Build history of the part. All positions in model axes, mm. Face numbers are marked on the shaded views. A direction names the side the tool comes from. Give positions to 0.01 mm unless a question says otherwise; leave off trailing zeros. Order: outer loops, then holes, each group sorted by start corner. A loop starts at its lowest first (then second) coordinate and runs counter-clockwise, first axis right, second up. Notation, with made-up numbers: (25.5, -31) - (77.5, -31) arc R17 ccw to (77.5, -26) - close; hole circle Ø5 at (19.25, 45.25). An arc over 180 degrees is marked (long way). Use a Markdown table: item, result.
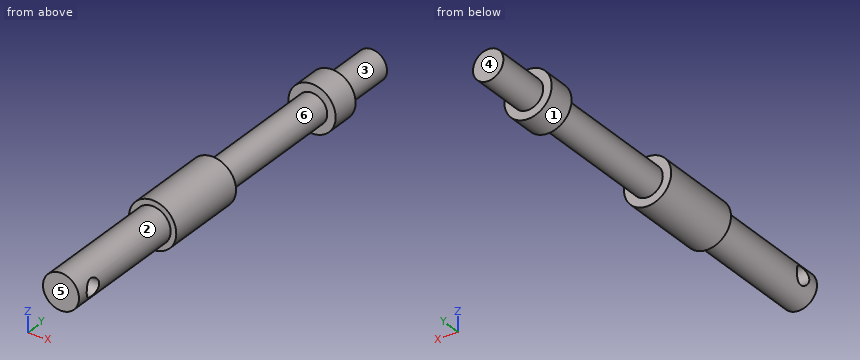
Autodesk Inventor part; units mm, degrees
ref_plane "YZ Plane" through (0, 0, 0) normal (1, 0, 0) x (0, 1, 0)
ref_plane "XZ Plane" through (0, 0, 0) normal (0, 1, 0) x (-1, 0, 0)
ref_plane "XY Plane" through (0, 0, 0) normal (0, 0, 1) x (1, 0, 0)
sketch "Sketch1" plane through (0, 0, 0) normal (1, 0, 0) x (0, 1, 0)
  line L0 (19.812, -0.0127) -> (0, -0.0127)
  line L1 (5.842, -0.8255) -> (5.842, -1.0795)
  line L2 (0, -0.0127) -> (0, -0.8255)
  line L3 (5.842, -0.8255) -> (0, -0.8255)
  line L4 (5.842, -1.0795) -> (9.652, -1.0795)
  line L5 (5.842, -1.0795) -> (9.652, -1.0795)
  line L6 (16.002, -1.0795) -> (17.272, -1.0795)
  line L7 (9.652, -1.0795) -> (9.652, -0.6985)
  line L8 (19.812, -0.6985) -> (17.272, -0.6985)
  line L9 (16.002, -0.6985) -> (9.652, -0.6985)
  line L10 (17.272, -1.0795) -> (17.272, -0.6985)
  line L11 (16.002, -0.6985) -> (16.002, -1.0795)
  line L12 (19.812, -0.0127) -> (19.812, -0.6985)
  line L13 (16.637, -1.0795) -> (16.637, -0.0127)
  line L14 (16.637, -0.0127) -> (0.889, -0.0127)
  circle A0 centre (0.889, -0.0127) radius 0.3969
  dimension "d9" = 0.8128
  dimension "d10" = 1.0668
  dimension "d11" = 0.6858
  dimension "d12" = 1.0668
  dimension "d13" = 0.6858
  dimension "d14" = 1.27
  dimension "d15" = 6.35
  dimension "d16" = 3.81
  dimension "d17" = 5.842
  dimension "d18" = 2.54
  dimension "d20" = 15.748
  dimension "d21" = 0.7937
revolve "Revolution1" add sketch "Sketch1" angle 360 about axis through (0, 19.812, -0.0127) along (0, -1, 0) picked at (1.1498, -0.0444) contours L12 L8 L10 L6 L13 L0 | L13 L6 L11 L9 L7 L4 L1 L3 L2 L0 A0 | A0 L0
extrude "Extrusion1" cut sketch "Sketch1" along normal mid plane 25.4 contours A0 L0 | L0 A0
properties part number "Valve"
1) Slice it at D-D (y = 2.25). Write the cut outline in (x, z).
Computed:
| item | result |
|---|---|
| outline | circle Ø1.63 at (0, -0.01) |
2) Slice it at B-B (x = -0.5). Write the cut outline in (y, z).
Computed:
| item | result |
|---|---|
| outline | (0, -0.65) - (5.84, -0.65) - (5.84, -0.96) - (9.65, -0.96) - (9.65, -0.48) - (16, -0.48) - (16, -0.96) - (17.27, -0.96) - (17.27, -0.48) - (19.81, -0.48) - (19.81, 0.46) - (17.27, 0.46) - (17.27, 0.93) - (16, 0.93) - (16, 0.46) - (9.65, 0.46) - (9.65, 0.93) - (5.84, 0.93) - (5.84, 0.63) - (0, 0.63) - close; hole circle Ø0.79 at (0.89, -0.01) |
3) Two-plate mould, pull along Y, no slides. Class the marked faces 3, 4, 5 and 6: +Y half, -Y half, draft (parallel to the pull), parting line (faces both ways), or undercut.
Computed:
| item | result |
|---|---|
| face 3 | draft |
| face 4 | +Y half |
| face 5 | -Y half |
| face 6 | undercut |
4) Wall check: line 1 (Y direction, x = -0.75, z = -0.2); line 2 (Y direction, x = 0.8, z = 0.5); line 3 (Y direction, x = -0.45, z = 0.6). Give the ranges that are in metal, low to high. Write a range as from..to.
Computed:
| item | result |
|---|---|
| line 1 | y = 0..0.54, 1.24..9.65, 16..17.27 |
| line 2 | y = 5.84..9.65, 16..17.27 |
| line 3 | y = 0..9.65, 16..17.27 |
5) Tool access for the marked faces 1 and 2: list every direction of +Z, -Z, +X, -X, +Y, -Y with a clear straight run to the whole face (end or side of a thin tool).
Computed:
| item | result |
|---|---|
| face 1 | +Y, -Y |
| face 2 | -Y |
6) Slice it at C-C (y = 7.5). Write the cut outline in (x, z), and give its area (3 significant figures).
Computed:
| item | result |
|---|---|
| outline | circle Ø2.13 at (0, -0.01) |
| area | 3.58 mm² |
7) Slice it at A-A (z = -0.2). Write the cut outline in (x, y).
Computed:
| item | result |
|---|---|
| outline | (-1.05, 5.84) - (-0.79, 5.84) - (-0.79, 1.24) - (0.79, 1.24) - (0.79, 5.84) - (1.05, 5.84) - (1.05, 9.65) - (0.66, 9.65) - (0.66, 16) - (1.05, 16) - (1.05, 17.27) - (0.66, 17.27) - (0.66, 19.81) - (-0.66, 19.81) - (-0.66, 17.27) - (-1.05, 17.27) - (-1.05, 16) - (-0.66, 16) - (-0.66, 9.65) - (-1.05, 9.65) - close; (-0.79, 0) - (0.79, 0) - (0.79, 0.54) - (-0.79, 0.54) - close |
